```python
from build123d import *

# Parameters (mm, degrees)
SKETCH3_W          = 35
SKETCH3_H          = 2
CHAMFER1_SIZE      = 0.6
CUT_EXTRUDE1_DEPTH = 1.61
SKETCH9_R          = 1.443375673
CUT_EXTRUDE2_DEPTH = 1.61
CUT_EXTRUDE2_DRAFT = -45


with BuildPart() as part:
    # Sketch3 → Revolve1 (revolve)
    with BuildSketch(Plane(origin=(0, 0, 0), x_dir=(0, 0, -1), z_dir=(1, 0, 0))):
        with Locations((0, 1)):
            Rectangle(SKETCH3_W, SKETCH3_H)
    revolve(axis=Axis((0, 0, -17.5), (0, 0, 1)))

    # Chamfer1
    chamfer1_edges = [part.edges().sort_by_distance(p)[0] for p in [
        (0, -2, -17.5),
    ]]
    chamfer(chamfer1_edges, length=CHAMFER1_SIZE)

    # Sketch6 → Revolve2 (revolve)
    with BuildSketch(Plane(origin=(0, 0, 0), x_dir=(0, 0, -1), z_dir=(1, 0, 0))):
        Polygon((-17.5, 4), (-17.2, 4), (-15.2, 2), (-15.2, 0), (-17.5, 0), align=None)
    revolve(axis=Axis((0, 0, -17.5), (0, 0, 1)))

    # Sketch8 → Cut-Extrude1 (cut)
    with BuildSketch(Plane.XY.offset(17.5)):
        Polygon((0, 1.443375673), (-1.25, 0.721687836), (-1.25, -0.721687836), (0, -1.443375673), (1.25, -0.721687836), (1.25, 0.721687836), align=None)
    extrude(amount=-CUT_EXTRUDE1_DEPTH, mode=Mode.SUBTRACT)


with BuildPart() as cut_extrude2_tool:
    # Sketch9 → Cut-Extrude2 (with draft: the straight prism first)
    with BuildSketch(Plane.XY.offset(17.5)):
        Circle(SKETCH9_R)
    extrude(amount=-CUT_EXTRUDE2_DEPTH)
    # Cut-Extrude2: the draft: its side faces are tilted about the plane it starts from
    cut_extrude2_sides = [cut_extrude2_tool.faces().sort_by_distance(p)[0] for p in [
        (-1.443375673, 0, 16.695),
    ]]
    draft(cut_extrude2_sides, Plane.XY.offset(17.5), CUT_EXTRUDE2_DRAFT)


with BuildPart() as part_1:
    add(part.part)

    # Cut-Extrude2: cut by cut_extrude2_tool
    add(cut_extrude2_tool.part, mode=Mode.SUBTRACT)


solid = part_1.part
```
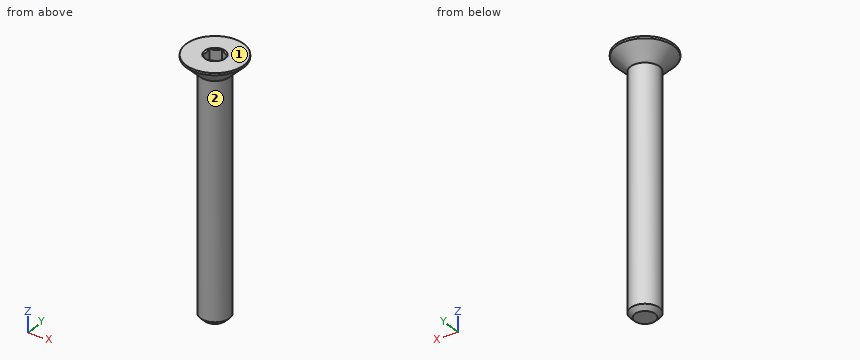
Here's how the part is built. I have some questions about the finished solid (model axes, mm). Face numbers are marked on the shaded views. A direction names the side the tool comes from. Give positions to 0.01 mm unless a question says otherwise; leave off trailing zeros. Write each loop counter-clockwise with the first axis right and the second up, starting at its lowest first coordinate (ties: lowest second). Pieces come first, ordered by that corner, then holes. Notation, with made-up numbers: (-3, 47) -> (5, 47) arc R22 cw to (5, 81) -> close; hole circle Ø3 at (51.5, 39.25). An arc over 180 degrees is marked (long way). Use one line per item in the form item = value.
1) Suppose I cut it at B-B (z = 6). Please give me the cut outline in (x, y), and give its area (3 significant figures).
Verdict:
outline = circle Ø4 at (0, 0)
area = 12.6 mm2
2) I'm going to push flat-ended pins straight in: pin 1 (4 mm diameter, centred on x = -0.5, z = 1, fed in from +Y); pin 2 (3 mm diameter, centred on x = -3, z = -8.5, fed in from +Y); pin 3 (2 mm diameter, centred on x = -3, y = 0.5, fed in from -Z). Where does each tip first touch, or does it pass through?
Verdict:
pin_1 = 2
pin_2 = 1.32
pin_3 = 15.24
3) If I drill on L1, parallel to X at y = 0, z = 2; L2, parallel to Z at x = 0.25, y = -0.5, over which ranges is the centre line in solid material (lowest first)? Write a range as [from, to].
Verdict:
L1 = [-2, 2]
L2 = [-17.5, 15.89]
4) On a 3-axis mill with a long thin cutter (end or side, diameter ignored), from which of +Z, -Z, +X, -X, +Y, -Y can I reach the whole of each face in a straight line? I mean the marked faces 1 and 2. Say none if no direction works.
Verdict:
face_1 = +Z, +X, -X, +Y, -Y
face_2 = -Z
5) Suppose I cut it at A-A (y = 0). Please give me the cut outline in (x, z), and give its area (3 significant figures).
Verdict:
outline = (-4, 17.2) -> (-2, 15.2) -> (-2, -16.9) -> (-1.4, -17.5) -> (1.4, -17.5) -> (2, -16.9) -> (2, 15.2) -> (4, 17.2) -> (4, 17.5) -> (1.44, 17.5) -> (1.25, 17.31) -> (1.25, 15.89) -> (-1.25, 15.89) -> (-1.25, 17.31) -> (-1.44, 17.5) -> (-4, 17.5) -> close
area = 141 mm2
